Autodesk Inventor part; units mm, degrees
ref_plane "YZ Plane" through (0, 0, 0) normal (1, 0, 0) x (0, 1, 0)
ref_plane "XZ Plane" through (0, 0, 0) normal (0, 1, 0) x (-1, 0, 0)
ref_plane "XY Plane" through (0, 0, 0) normal (0, 0, 1) x (1, 0, 0)
sketch "Sketch1" plane through (0, 0, 0) normal (0, 0, 1) x (1, 0, 0)
  line L0 (-110.5, 0) -> (110.5, 0) construction
  line L1 (0, 110.5) -> (0, -110.5) construction
  line L2 (-110.5, 110.5) -> (110.5, 110.5) construction
  line L3 (110.5, 110.5) -> (110.5, -110.5) construction
  line L4 (110.5, -110.5) -> (-110.5, -110.5) construction
  line L5 (-110.5, -110.5) -> (-110.5, 110.5) construction
  circle A0 centre (-37.5, 0) radius 37.5 construction
  circle A1 centre (37.5, 0) radius 37.5 construction
  arc A2 (-2.1447, 35.3553) -> (-87.5, 0) centre (-37.5, 0) ccw
  arc A3 (-2.1447, 35.3553) -> (0, 34.467) centre (0, 37.5) ccw
  line L6 (-37.5, 0) -> (-2.1447, 35.3553) construction
  arc A4 (-47.5716, 57.1188) -> (-74.8373, 44.3838) centre (-37.5, 0) ccw
  arc A5 (-12.404, 52.2895) -> (-27.5, 57.1314) centre (-37.5, 0) ccw
  arc A6 (-12.404, 52.2895) -> (0, 49.467) centre (0, 78.1341) ccw
  line L7 (-37.5, 0) -> (-110.5, 61.2543) construction
  line L8 (-37.5, 0) -> (20.5, 0) construction
  line L9 (-37.5, 0) -> (-37.5, 110.5) construction
  line L10 (-87.6931, 29.0629) -> (-99.8491, 39.2631)
  arc A7 (-86.9934, 54.5839) -> (-99.8491, 39.2631) centre (-93.4212, 46.9235) ccw
  line L11 (-86.9934, 54.5839) -> (-74.8373, 44.3838)
  circle A8 centre (-93.4212, 46.9235) radius 3.3
  line L12 (-97.844, 50.6346) -> (-92.4187, 52.6093) construction
  line L13 (-92.4187, 52.6093) -> (-87.9959, 48.8981) construction
  line L14 (-87.9959, 48.8981) -> (-88.9985, 43.2124) construction
  line L15 (-88.9985, 43.2124) -> (-94.4238, 41.2377) construction
  line L16 (-94.4238, 41.2377) -> (-98.8466, 44.9488) construction
  line L17 (-98.8466, 44.9488) -> (-97.844, 50.6346) construction
  line L18 (-47.5, 57.1314) -> (-47.5, 73)
  line L19 (-27.5, 73) -> (-27.5, 57.1314)
  line L20 (-32.5, 70.1132) -> (-37.5, 67.2265) construction
  line L21 (-37.5, 78.7735) -> (-32.5, 75.8868) construction
  line L22 (-37.5, 67.2265) -> (-42.5, 70.1132) construction
  line L23 (-42.5, 75.8868) -> (-37.5, 78.7735) construction
  arc A9 (-27.5, 73) -> (-47.5, 73) centre (-37.5, 73) ccw
  line L24 (-32.5, 75.8868) -> (-32.5, 70.1132) construction
  circle A10 centre (-37.5, 73) radius 3.3
  line L25 (-42.5, 70.1132) -> (-42.5, 75.8868) construction
  line L26 (-37.5, 0) -> (-2.1447, -35.3553) construction
  line L27 (0, 49.467) -> (0, 34.467)
  arc A11 (-27.5, 57.1314) -> (-47.5, 57.1314) centre (-37.5, 0) ccw construction
  arc A12 (-47.5, 57.1314) -> (-47.5716, 57.1188) centre (-37.5, 0) ccw
  arc A13 (-74.8373, 44.3838) -> (-87.6931, 29.0629) centre (-37.5, 0) ccw construction
  arc A14 (-87.6931, 29.0629) -> (-95.5, 0) centre (-37.5, 0) ccw
  line L28 (-95.5, 0) -> (-87.5, 0)
  point P0 (0, 0)
  point P1 (0, 0)
  point P2 (0, 0)
  point P3 (-81.9306, 37.2817)
  point P4 (-37.5, 58)
  dimension "d10" = 75
  dimension "d7" = 221
  dimension "d8" = 221
  dimension "d9" = 75
  dimension "d11" = 50
  dimension "d12" = 135
  dimension "d13" = 8
  dimension "d14" = 15
  dimension "d15" = 140
  dimension "d17" = 10
  dimension "d19" = 6.6
  dimension "d20" = 15
  dimension "d21" = 10
  dimension "d24" = 50
extrude "Extrusion1" add sketch "Sketch1" along normal blind 50
sketch "Sketch4" plane through (0, 0, 50) normal (0, 0, 1) x (1, 0, 0)
  line L0 (0, 0) -> (0, 122) construction
  line L1 (0, 0) -> (-181, 0) construction
  arc A0 (-87.6931, 29.0629) -> (-95.5, 0) centre (-37.5, 0) ccw construction
  arc A1 (-12.404, 52.2895) -> (-95.5, 0) centre (-37.5, 0) ccw
  arc A2 (-12.404, 52.2895) -> (0, 49.467) centre (0, 78.1341) ccw
  line L2 (0, 49.467) -> (0, 0)
  arc A3 (-87.6931, 29.0629) -> (-95.5, 0) centre (-37.5, 0) ccw
sketch "Sketch5" plane through (0, 34.467, 0) normal (1, 0, 0) x (0, 0, -1)
  arc A0 (-50, 23.533) -> (-66, -34.467) centre (47.125, -34.467) ccw
  line L0 (-50, -34.467) -> (-50, 15.533) construction
  line L1 (-50, -34.467) -> (-94, -34.467) construction
  line L2 (0, -34.467) -> (-50, -34.467) construction
  line L3 (-50, 22.6644) -> (-50, 38.533)
  dimension "d28" = 116
  dimension "d29" = 16
equation "\"d10\" = d9"
properties part number "Gehäuse"
Can you work these out from the model? Positions are in its coordinate system, mm. A direction names the side the tool comes from. Give positions to 0.01 mm unless a question says otherwise; leave off trailing zeros. Order: outer loops, then holes, each group sorted by start corner. A loop starts at its lowest first (then second) coordinate and runs counter-clockwise, first axis right, second up. Notation, with made-up numbers: M 3,-2 L 23,-2 A25 cw 23,26 Z; hole C 86,56.5 d8. An arc over 180 degrees is marked long. One line per item, written item: value.
Item 1: If we section it at B-B on z = 16.5: Write out the boundary of the cut face in (x, y).
Verdict:
outline: M -99.85,39.26 L -87.69,29.06 A58 ccw -95.5,0 L -87.5,0 A50 cw -2.14,35.36 A3.03 ccw 0,34.47 L 0,49.47 A28.67 cw -12.4,52.29 A58 ccw -27.5,57.13 L -27.5,73 A10 ccw -47.5,73 L -47.5,57.13 A30.24 ccw -47.57,57.12 A58 ccw -74.84,44.38 L -86.99,54.58 A10 ccw Z; hole C -93.42,46.92 d6.6; hole C -37.5,73 d6.6
Item 2: If we section it at A-A on x = -37.5: Write out the boundary of the cut face in (y, z).
Verdict:
outline: M 50,0 L 69.7,0 L 69.7,50 L 50,50 Z; M 76.3,0 L 83,0 L 83,50 L 76.3,50 Z
Item 3: If we section it at C-C on y = 26: Write out the boundary of the cut face in (x, z).
Verdict:
outline: M -89.35,0 L -80.21,0 L -80.21,50 L -89.35,50 Z
Item 4: For faces 1 (the face through (-62.24, 52.46, 24.65)), 2 (the face through (-1.145, 34.691, 24.65)), 3 (the face through (-93.57, 14.84, 24.65)), 4 (the face through (-47.5, 65, 25)), which set-ups out of +Z, -Z, +X, -X, +Y, -Y let a thin tool reach every point of the face, with its end or its side?
Verdict:
face 1: +Z, -Z, +Y
face 2: +Z, -Z, -Y
face 3: +Z, -Z, -X
face 4: +Z, -Z, -X, +Y
Item 5: If we section it at D-D on x = -66: Write out the boundary of the cut face in (y, z), and give its area (3 significant figures).
Verdict:
outline: M 41.08,0 L 50.51,0 L 50.51,50 L 41.08,50 Z
area: 472 mm2
Item 6: For pin 1 (8 mm diameter, centred on y = 63.5, z = 34.5, fed in from -X); pin 2 (3 mm diameter, centred on y = 9, z = 28.5, fed in from -X); pin 3 (5.5 mm diameter, centred on x = -93.42, y = 46.92, fed in from +Z); pin 4 (6 mm diameter, centred on x = -85.5, z = 19.5, fed in from +Y), each with a flat end and sliding along its axis, tell me the tip position at first contact or that it passes through.
Verdict:
pin 1: x = -47.5
pin 2: x = -95.01
pin 3: through
pin 4: y = 55.63
Item 7: Please list where these lines run through material, in increasing order: line 1 (Y direction, x = -37.5, z = 23); line 2 (X direction, y = 39.5, z = 9); line 3 (X direction, y = 65, z = 32).
Verdict:
line 1: 50 to 69.7, 76.3 to 83
line 2: -100.12 to -68.16, -6.84 to 0
line 3: -47.5 to -27.5
Item 8: If we mould it in two halves opening along Y, with no side actions, what happens to faces 5 (the face through (-56, 48, 50)), 6 (the face through (-19.89, 55.26, 24.65)), 7 (the face through (-93.686, 34.092, 24.65)), 8 (the face through (-96.72, 46.78, 24.65))? For each: pulls with the +Y half, pulls with the -Y half, needs draft (parallel to the pull), parting line crosses it, or undercut.
Verdict:
face 5: needs draft
face 6: pulls with the +Y half
face 7: undercut
face 8: undercut
